from build123d import *

# Parameters (mm, degrees)
F1_DEPTH = 650
F2_R     = 10
F3_DEPTH = 25


with BuildPart() as f1:
    # F0 (on Front) → F1 (new body, symmetric)
    with BuildSketch(Plane.XZ):
        with BuildLine():
            Line((19, 25), (-19, 25))
            ThreePointArc((-19, 25), (-23.242641, 23.242641), (-25, 19))
            Line((-25, 19), (-25, -19))
            ThreePointArc((-25, -19), (-23.242641, -23.242641), (-19, -25))
            Line((-19, -25), (19, -25))
            ThreePointArc((19, -25), (23.242641, -23.242641), (25, -19))
            Line((25, -19), (25, 19))
            ThreePointArc((25, 19), (23.242641, 23.242641), (19, 25))
        make_face()
        with BuildLine():
            ThreePointArc((-21, 19), (-20.414214, 20.414214), (-19, 21))
            Line((-19, 21), (19, 21))
            ThreePointArc((19, 21), (20.414214, 20.414214), (21, 19))
            Line((21, 19), (21, -19))
            ThreePointArc((21, -19), (20.414214, -20.414214), (19, -21))
            Line((19, -21), (-19, -21))
            ThreePointArc((-19, -21), (-20.414214, -20.414214), (-21, -19))
            Line((-21, -19), (-21, 19))
        make_face(mode=Mode.SUBTRACT)
    extrude(amount=F1_DEPTH, both=True)

    # F2 (on face) → F3 (cut)
    with BuildSketch(Plane.XY.offset(25)):
        with Locations((0, -450)):
            Circle(F2_R)
    extrude(amount=-F3_DEPTH, mode=Mode.SUBTRACT)


solid = f1.part
Input: part model. Units: mm. Frame: model coordinates. A direction names the side the tool comes from. Round coordinates to 2 decimals unless told otherwise and drop trailing zeros. Loops run counter-clockwise (first coordinate to the right, second up) from the corner with the lowest first, then second, coordinate; pieces in that order, holes last. Notation, with made-up numbers: (-8, -39.75) -> (45, -39.75) arc R25 cw to (45, -18.75) -> close; hole circle Ø4 at (-34, 84.25). An arc over 180 degrees is marked (long way). Answer as a JSON object with one key per item and string values. Group by question number.
1) Ray query, L1, parallel to Z at x = 1.5, y = 415; L2, parallel to Y at x = 0, z = 24.1. Return the intervals inside material, ascending.
2) Section query A-A on z = 6.5. Output: boundary loops of the cut face in (x, y).
3) Section query B-B on x = 0. Output: boundary loops of the cut face in (y, z).
4) Pin query (flat end, axial travel): pin 1 (2 mm diameter, centred on x = 19.5, z = -7.5, fed in from -Y). Return the tip coordinate at first contact, or that it passes through.
5) Draft query along Z for faces 1 (the flat face through (0, -9, 21)), 2 (the flat face through (0, -9, -25)), 3 (the flat face through (25, -9, 0)). Return one class per face: +Z half, -Z half, draft (parallel to the pull), parting line (faces both ways), or undercut.
6) Section query C-C on y = 563. Output: boundary loops of the cut face in (x, z).
7) Reachability of faces 4 (the flat face through (-23, 650, 0)), 5 (the cylindrical face through (-1.302, -440.085, 23.028)), 6 (the flat face through (21, -9, 0)) from +Z, -Z, +X, -X, +Y, -Y: full face, straight path, thin tool, end or side. Return the list, or none.
Reply:
{
 "1": {"L1": "z = -25 to -21, 21 to 25", "L2": "y = -650 to -460, -440 to 650"},
 "2": {"outline": "(-25, -650) -> (-21, -650) -> (-21, 650) -> (-25, 650) -> close; (21, -650) -> (25, -650) -> (25, 650) -> (21, 650) -> close"},
 "3": {"outline": "(-650, -25) -> (650, -25) -> (650, -21) -> (-650, -21) -> close; (-650, 21) -> (-460, 21) -> (-460, 25) -> (-650, 25) -> close; (-440, 21) -> (650, 21) -> (650, 25) -> (-440, 25) -> close"},
 "4": {"pin 1": "passes through"},
 "5": {"face 1": "undercut", "face 2": "-Z half", "face 3": "draft"},
 "6": {"outline": "(-25, -19) arc R6 ccw to (-19, -25) -> (19, -25) arc R6 ccw to (25, -19) -> (25, 19) arc R6 ccw to (19, 25) -> (-19, 25) arc R6 ccw to (-25, 19) -> close; hole (-21, -19) arc R2 ccw to (-19, -21) -> (19, -21) arc R2 ccw to (21, -19) -> (21, 19) arc R2 ccw to (19, 21) -> (-19, 21) arc R2 ccw to (-21, 19) -> close"},
 "7": {"face 4": "+Z, -Z, +X, -X, +Y", "face 5": "+Z", "face 6": "+Y, -Y"}
}
